Geometry: see drawing. Coordinates: mm, zero at the bounding-box minimum. Give positions to 0.01 mm unless a question says otherwise; leave off trailing zeros. Order: outer loops, then holes, each group sorted by start corner. A loop starts at its lowest first (then second) coordinate and runs counter-clockwise, first axis right, second up. Notation, with made-up numbers: (-27, 88) - (-3, 88) arc R33 cw to (-3, 126) - close; hole circle Ø1 at (-8.5, -38.5). An arc over 180 degrees is marked (long way). Write each question's results on one line, items separated by ' | '. Start each with the question number.
Item 1: Section B-B on y = 2.65. Output: boundary loops of the cut face in (x, z) (1 decimal), and give its area (3 significant figures).
Item 2: Line query: line 1 along Z through (x, y) = (19.5, 1) (1 decimal); line 2 along Z through (x, y) = (44, 2.85) (1 decimal); line 3 along Z through (x, y) = (58, 2) (1 decimal). Output: solid intervals per line, ascending.
Item 3: Section A-A on x = 45. Output: boundary loops of the cut face in (y, z), and give its area (3 significant figures).
Item 4: Contact query for a flat-ended pin moving along its axis: pin 1 Ø2 at (x, y) = (45, 2.5) entering from +Z. Output: stop coordinate, or through.
Item 5: Section D-D on x = 29. Output: boundary loops of the cut face in (y, z).
Item 6: Section C-C on z = 72. Output: boundary loops of the cut face in (x, y), and give its area (3 significant figures).
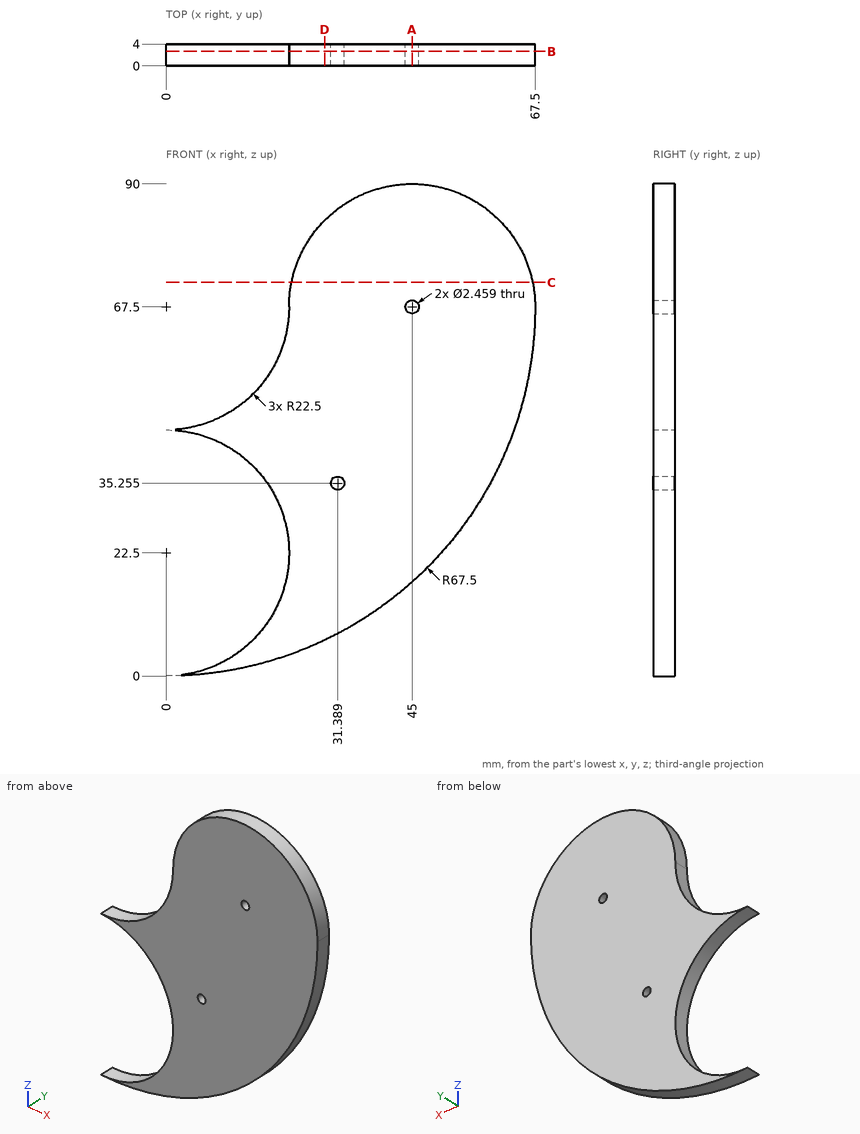
Evaluation:
1) outline: (0, 0) arc R67.5 ccw to (67.5, 67.5) arc R22.5 ccw to (22.5, 67.5) arc R22.5 cw to (0, 45) arc R22.5 cw to start; hole circle Ø2.5 at (31.4, 35.3); hole circle Ø2.5 at (45, 67.5) | area: 3,170 mm^2
2) line 1: z = 2.9 to 11.3, 33.7 to 56.3 | line 2: z = 16.3 to 66.8, 68.2 to 90 | line 3: z = 33 to 85.9
3) outline: (0, 17.19) - (4, 17.19) - (4, 66.27) - (0, 66.27) - close; (0, 68.73) - (4, 68.73) - (4, 90) - (0, 90) - close | area: 281 mm^2
4) pin 1: stops at z = 90
5) outline: (0, 6.55) - (4, 6.55) - (4, 83.32) - (0, 83.32) - close
6) outline: (22.95, 0) - (67.05, 0) - (67.05, 4) - (22.95, 4) - close | area: 176 mm^2
